Part print with two shaded views. Sizes in mm from the minimum x, y, z corner. Round coordinates to 2 decimals unless told otherwise and drop trailing zeros. Write each loop counter-clockwise with the first axis right and the second up, starting at its lowest first coordinate (ties: lowest second). Pieces come first, ordered by that corner, then holes. Notation, with made-up numbers: (2, 8.5) -> (25, 8.5) arc R6 ccw to (25, 13.5) -> close; hole circle Ø1 at (57.5, 40). An arc over 180 degrees is marked (long way). Answer as CSV lines item,"result".
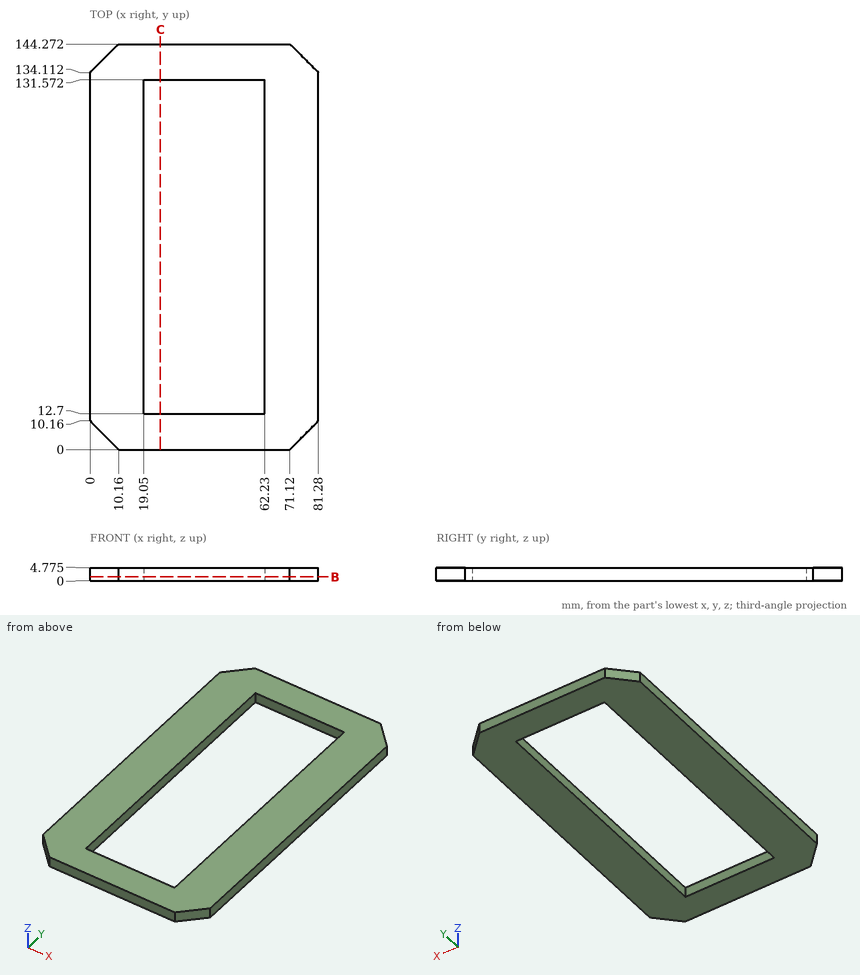
1. Cut at B-B, the plane z = 1.45. Write the cut outline in (x, y).
Results found:
outline,"(0, 10.16) -> (10.16, 0) -> (71.12, 0) -> (81.28, 10.16) -> (81.28, 134.11) -> (71.12, 144.27) -> (10.16, 144.27) -> (0, 134.11) -> close; hole (19.05, 12.7) -> (62.23, 12.7) -> (62.23, 131.57) -> (19.05, 131.57) -> close"
2. Probe line 1 along X through (y, z) = (127, 3.4); line 2 along Y through (x, z) = (27, 3.35); line 3 along X through (y, z) = (136, 2.4). List the from-to ranges inside material, lowest first.
Results found:
line 1,"x = 0 to 19.05, 62.23 to 81.28"
line 2,"y = 0 to 12.7, 131.57 to 144.27"
line 3,"x = 1.89 to 79.39"
3. Cut at C-C, the plane x = 25. Write the cut outline in (y, z) (1 decimal), then the cut area to 3 significant figures.
Results found:
outline,"(0, 0) -> (12.7, 0) -> (12.7, 4.8) -> (0, 4.8) -> close; (131.6, 0) -> (144.3, 0) -> (144.3, 4.8) -> (131.6, 4.8) -> close"
area,"121 mm2"
